The listing builds one solid part. Answer for the finished solid, in the listing's coordinates (mm). A direction names the side the tool comes from. Round coordinates to 2 decimals unless told otherwise and drop trailing zeros. Write each loop counter-clockwise with the first axis right and the second up, starting at its lowest first coordinate (ties: lowest second). Pieces come first, ordered by that corner, then holes.
Item 1: Each of these flat-tipped pins is pushed along its axis until it touches: pin 1 (3.5 mm diameter, centred on y = 2, z = 17.5, fed in from +X); pin 2 (2.5 mm diameter, centred on y = 22.5, z = 14, fed in from +X); pin 3 (1.8 mm diameter, centred on x = 14, z = 19.5, fed in from -Y). Where does it stop, or does it pass through?
Item 2: Find section C-C on y = 17.75. Give the vertices of the cut face in (x, z).
Item 3: Find the intervals of material crossed by probe 1 along Z at (x, y) = (7.5, 19.5); probe 2 along X at (y, z) = (23, 16.5); probe 3 along Y at (x, z) = (8.5, 3.2), in increasing order.
Item 4: Find section D-D on x = 14.25. Give the vertices of the cut face in (y, z), then the cut area to 3 significant figures.
Item 5: A tool of negligible diameter and unlimited length cuts with its end or side. For faces 5 (the face through (13.247, 13.199, 18.215)), 6 (the face through (1.5, 22, 14)), 7 (the face through (13.093, 3.601, 0.285)), from which of +Z, -Z, +X, -X, +Y, -Y can it reach the whole face along a straight path? Write none if from no direction.
Item 6: Find section A-A on y = 10. Give the vertices of the cut face in (x, z).
Item 7: Find section B-B on z = 3.2. Give the vertices of the cut face in (x, y).
Item 8: For a pull along Y with two mould halves and no side action, classify faces 1 (the face through (6, 16, 18.5)), 2 (the face through (1.585, 6.801, 13.951)), 3 (the face through (7, 15, 28)), 4 (the face through (13, 16.7, 14)) as +Y half, -Y half, draft (parallel to the pull), parting line (faces both ways), or undercut.
```python
from build123d import *

# Parameters (mm, degrees)
EXTRUDE_1_DEPTH          = 28
SKETCH_2_R               = 1.6
CUT_EXTRUDE_1_DEPTH      = 1
CUT_EXTRUDE_1_DEPTH_BACK = 18.1
SKETCH_4_W               = 9
SKETCH_4_H               = 7
CUT_EXTRUDE_2_DEPTH      = 15.8
SKETCH_5_W               = 7
SKETCH_5_H               = 9
CUT_EXTRUDE_3_DEPTH      = 23
FILLET_1_R               = 1.5
FILLET_2_R               = 1
FILLET_3_R               = 1


with BuildPart() as part:
    # 草图1 → 凸台-拉伸1 (new body)
    with BuildSketch(Plane.XY):
        Polygon((0, 30), (0, 0), (10, 0), (10, 3.3), (17.1, 3.3), (17.1, 16.7), (10, 16.7), (10, 30), align=None)
    extrude(amount=EXTRUDE_1_DEPTH)

    # 草图2 → 切除-拉伸1 (cut, two sides)
    with BuildSketch(Plane(origin=(17.1, 0, 0), x_dir=(0, 0, -1), z_dir=(1, 0, 0))) as cut_extrude_1_sk:
        with Locations((-24.8, 10)):
            Circle(SKETCH_2_R)
        with Locations((-3.2, 10)):
            Circle(SKETCH_2_R)
    extrude(amount=CUT_EXTRUDE_1_DEPTH, mode=Mode.SUBTRACT)
    extrude(cut_extrude_1_sk.sketch, amount=-CUT_EXTRUDE_1_DEPTH_BACK, mode=Mode.SUBTRACT)

    # 草图4 → 切除-拉伸2 (cut)
    with BuildSketch(Plane(origin=(17.1, 0, 0), x_dir=(0, 0, -1), z_dir=(1, 0, 0))):
        with Locations((-14, 10)):
            Rectangle(SKETCH_4_W, SKETCH_4_H)
    extrude(amount=-CUT_EXTRUDE_2_DEPTH, mode=Mode.SUBTRACT)

    # 草图5 → 切除-拉伸3 (cut)
    with BuildSketch(Plane(origin=(0, 30, 0), x_dir=(1, 0, 0), z_dir=(0, 1, 0))):
        with Locations((5, -14)):
            Rectangle(SKETCH_5_W, SKETCH_5_H)
    extrude(amount=-CUT_EXTRUDE_3_DEPTH, mode=Mode.SUBTRACT)

    # 圆角1
    fillet_1_edges = [part.edges().sort_by_distance(p)[0] for p in [
        (0, 15, 0),
        (0, 15, 28),
    ]]
    fillet(fillet_1_edges, radius=FILLET_1_R)

    # 圆角2
    fillet_2_edges = [part.edges().sort_by_distance(p)[0] for p in [
        (8.5, 13.5, 14),
        (8.5, 21.75, 18.5),
        (8.5, 21.75, 9.5),
        (12.8, 13.5, 18.5),
        (12.8, 13.5, 9.5),
        (9.2, 6.5, 9.5),
        (9.2, 6.5, 18.5),
        (1.3, 6.5, 14),
        (1.3, 10, 18.5),
        (1.3, 10, 9.5),
    ]]
    fillet(fillet_2_edges, radius=FILLET_2_R)

    # 圆角3
    fillet_3_edges = [part.edges().sort_by_distance(p)[0] for p in [
        (17.1, 16.7, 14),
        (17.1, 3.3, 14),
        (13.55, 3.3, 28),
        (17.1, 10, 28),
        (13.55, 16.7, 28),
        (13.55, 16.7, 0),
        (17.1, 10, 0),
        (13.55, 3.3, 0),
    ]]
    fillet(fillet_3_edges, radius=FILLET_3_R)


solid = part.part
```
Check values:
1. pin 1: stops at x = 16.94
1. pin 2: stops at x = 10
1. pin 3: stops at y = 3.3
2. outline: (0, 1.5) arc R1.5 ccw to (1.5, 0) - (10, 0) - (10, 28) - (1.5, 28) arc R1.5 ccw to (0, 26.5) - close; hole (1.5, 9.9) arc R1 ccw to (2.3, 9.5) - (7.5, 9.5) arc R1 ccw to (8.5, 10.5) - (8.5, 17.5) arc R1 ccw to (7.5, 18.5) - (2.3, 18.5) arc R1 ccw to (1.5, 18.1) - close
3. probe 1: z = 0 to 9.5, 18.5 to 28
3. probe 2: x = 0 to 1.5, 8.5 to 10
3. probe 3: y = 0 to 8.4, 11.6 to 30
4. outline: (3.3, 1) arc R1 ccw to (4.3, 0) - (15.7, 0) arc R1 ccw to (16.7, 1) - (16.7, 27) arc R1 ccw to (15.7, 28) - (4.3, 28) arc R1 ccw to (3.3, 27) - close; hole (6.5, 10.5) arc R1 ccw to (7.5, 9.5) - (12.5, 9.5) arc R1 ccw to (13.5, 10.5) - (13.5, 17.5) arc R1 ccw to (12.5, 18.5) - (7.5, 18.5) arc R1 ccw to (6.5, 17.5) - close; hole circle Ø3.2 at (10, 3.2); hole circle Ø3.2 at (10, 24.8)
4. area: 296 mm2
5. face 5: +X
5. face 6: +Y
5. face 7: -Z, +X, -Y
6. outline: (0, 1.5) arc R1.5 ccw to (1.5, 0) - (16.1, 0) arc R1 ccw to (17.1, 1) - (17.1, 1.6) - (0, 1.6) - close; (0, 4.8) - (17.1, 4.8) - (17.1, 9.5) - (2.3, 9.5) arc R1 cw to (1.3, 10.5) - (1.3, 17.5) arc R1 cw to (2.3, 18.5) - (17.1, 18.5) - (17.1, 23.2) - (0, 23.2) - close; (0, 26.4) - (17.1, 26.4) - (17.1, 27) arc R1 ccw to (16.1, 28) - (1.5, 28) arc R1.5 ccw to (0, 26.5) - close
7. outline: (0, 0) - (10, 0) - (10, 3.3) - (16.1, 3.3) arc R1 ccw to (17.1, 4.3) - (17.1, 8.4) - (0, 8.4) - close; (0, 11.6) - (17.1, 11.6) - (17.1, 15.7) arc R1 ccw to (16.1, 16.7) - (10, 16.7) - (10, 30) - (0, 30) - close
8. face 1: undercut
8. face 2: undercut
8. face 3: draft
8. face 4: +Y half
